from build123d import *

# Parameters (mm, degrees)
SKETCH_1_W          = 92
SKETCH_1_H          = 190
EXTRUDE_1_DEPTH     = 3
SKETCH_2_R          = 1.5
CUT_EXTRUDE_1_DEPTH = 106.59356041
CUT_EXTRUDE_2_DEPTH = 106.59356041
FILLET_2_R          = 2


with BuildPart() as part:
    # 草图1 → 凸台-拉伸1 (new body)
    with BuildSketch(Plane.XY):
        Rectangle(SKETCH_1_W, SKETCH_1_H)
    extrude(amount=EXTRUDE_1_DEPTH)

    # 草图2 → 切除-拉伸1 (cut, through all)
    with BuildSketch(Plane.XY.offset(3)):
        with Locations((-34, 87.5)):
            Circle(SKETCH_2_R)
        with Locations((16, 87.5)):
            Circle(SKETCH_2_R)
        with Locations((38.5, 65)):
            Circle(SKETCH_2_R)
        with Locations((38.5, -55)):
            Circle(SKETCH_2_R)
    extrude(amount=-CUT_EXTRUDE_1_DEPTH, mode=Mode.SUBTRACT)

    # 草图3 → 切除-拉伸2 (cut, through all)
    with BuildSketch(Plane.XY.offset(3)):
        Polygon((19, -15), (16, -15), (-31, -77), (-31, -85), (19, -85), align=None)
    extrude(amount=-CUT_EXTRUDE_2_DEPTH, mode=Mode.SUBTRACT)

    # 圆角2
    fillet_2_edges = [part.edges().sort_by_distance(p)[0] for p in [
        (-31, -77, 1.5),
        (16, -15, 1.5),
        (19, -15, 1.5),
        (19, -85, 1.5),
        (-31, -85, 1.5),
    ]]
    fillet(fillet_2_edges, radius=FILLET_2_R)


solid = part.part
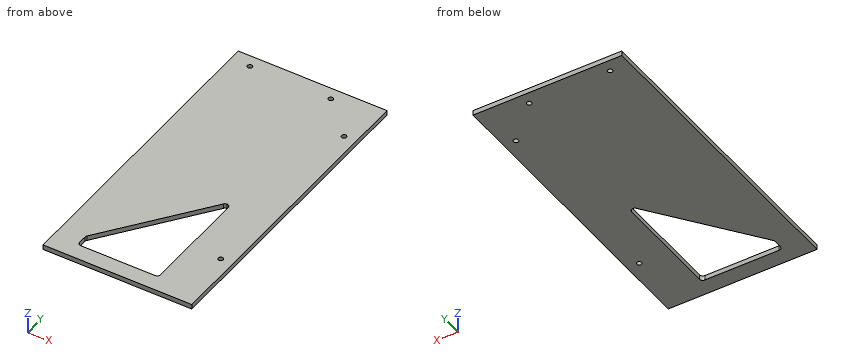
Check sheet for the modelled part. Datum: model origin and axes. Units: mm. Give positions to 0.01 mm unless a question says otherwise; leave off trailing zeros. Write each loop counter-clockwise with the first axis right and the second up, starting at its lowest first coordinate (ties: lowest second). Pieces come first, ordered by that corner, then holes. Notation, with made-up numbers: (-6, -16.5) -> (42, -16.5) arc R32 cw to (42, 14.5) -> close; hole circle Ø4 at (84.25, 34.25). An arc over 180 degrees is marked (long way). Write item = value, one per line.
Item 1: Sectioned sample at C-C on y = -27.5. Record the boundary of the cut face in (x, z).
Output:
outline = (-46, 0) -> (6.52, 0) -> (6.52, 3) -> (-46, 3) -> close; (19, 0) -> (46, 0) -> (46, 3) -> (19, 3) -> close
Item 2: Sectioned sample at A-A on z = 2.4. Count the separate pieces of the cut face and the enclosed holes in it, and give its area (3 significant figures).
Output:
separate_pieces = 1
enclosed_holes = 5
area = 15,400 mm^2
Item 3: Sectioned sample at B-B on x = 0. Record the boundary of the cut face in (y, z).
Output:
outline = (-95, 0) -> (-85, 0) -> (-85, 3) -> (-95, 3) -> close; (-36.11, 0) -> (95, 0) -> (95, 3) -> (-36.11, 3) -> close
Item 4: Scan lines: probe 1 along Y at (x, z) = (38.5, 1); probe 2 along X at (y, z) = (87.5, 1.8); probe 3 along Y at (x, z) = (16, 1.45). Record each from-to range of solid material in increasing order. Write a range as from..to.
Output:
probe_1 = -95..-56.5, -53.5..63.5, 66.5..95
probe_2 = -46..-35.5, -32.5..14.5, 17.5..46
probe_3 = -95..-85, -15.26..86, 89..95
Item 5: Gauge pin test, flat end, axial feed: pin 1 (1.8 mm diameter, centred on x = 16, y = 87.5, fed in from -Z). Record the tip position at first contact, or that the pin passes through.
Output:
pin_1 = through
